from build123d import *

# Parameters (mm, degrees)
F1_DEPTH = 12.7
F3_DEPTH = 12.7
F5_D     = 16.002


with BuildPart() as f1:
    # F0 (on Front) → F1 (new body)
    with BuildSketch(Plane.XZ):
        with BuildLine():
            Line((0, 69.85), (0, 0))
            Line((0, 0), (15.67386, 0))
            Line((15.67386, 0), (16.004092, 12.86297))
            ThreePointArc((16.004092, 12.86297), (21.769188, 19.023198), (28.563172, 14.020547))
            ThreePointArc((28.563172, 14.020547), (28.702, 12.7), (28.563172, 11.379453))
            Line((28.563172, 11.379453), (28.563172, 0))
            Line((28.563172, 0), (44.704, 0))
            Line((44.704, 0), (44.704, 69.85))
            ThreePointArc((44.704, 69.85), (22.352, 92.202), (0, 69.85))
        make_face()
    extrude(amount=F1_DEPTH)

    # F2 (on face) → F3 (join)
    with BuildSketch(Plane.XZ.offset(12.7)):
        with BuildLine():
            Line((0, 69.85), (0, 44.45))
            Line((0, 44.45), (2.100821, 44.45))
            Line((2.100821, 44.45), (44.704, 44.45))
            Line((44.704, 44.45), (44.704, 69.85))
            ThreePointArc((44.704, 69.85), (22.352, 92.202), (0, 69.85))
        make_face()
    extrude(amount=F3_DEPTH)

    # F5 (through all)
    with Locations(Plane.XZ.offset(25.4)):
        with Locations((22.352, 69.85)):
            Hole(F5_D / 2)


solid = f1.part
Could you check a few things on this model? Use its own coordinates, in mm. A direction names the side the tool comes from. Round coordinates to 2 decimals unless told otherwise and drop trailing zeros. Order: outer loops, then holes, each group sorted by start corner. A loop starts at its lowest first (then second) coordinate and runs counter-clockwise, first axis right, second up.
(1) If we mould it in two halves opening along X, with no side actions, what happens to faces 1 (the flat face through (17, -25.4, 63)), 2 (the flat face through (0, -10, 43)), 3 (the flat face through (28.563, -6, 6))? For each: released by +X, released by -X, zero draft, split by the parting line, or undercut.
Response values:
face 1: zero draft
face 2: released by -X
face 3: undercut
(2) Imagine slicing it at A-A (z = 72). Write out the boundary of the cut face in (x, y), plus the area to 3 significant figures.
Response values:
outline: (0.1, -25.4) - (14.65, -25.4) - (14.65, 0) - (0.1, 0) - close; (30.06, -25.4) - (44.6, -25.4) - (44.6, 0) - (30.06, 0) - close
area: 739 mm2
(3) Imagine slicing it at D-D (y = -14.5). Write out the boundary of the cut face in (x, z).
Response values:
outline: (0, 44.45) - (44.7, 44.45) - (44.7, 69.85) arc R22.35 ccw to (0, 69.85) - close; hole circle Ø16 at (22.35, 69.85)
(4) Imagine slicing it at B-B (y = -6.5). Write out the boundary of the cut face in (x, z).
Response values:
outline: (0, 0) - (15.67, 0) - (16, 12.86) arc R6.35 cw to (28.56, 14.02) arc R6.35 cw to (28.56, 11.38) - (28.56, 0) - (44.7, 0) - (44.7, 69.85) arc R22.35 ccw to (0, 69.85) - close; hole circle Ø16 at (22.35, 69.85)
(5) I'm going to push flat-ended pins straight in: pin 1 (3 mm diameter, centred on x = 17, y = -14, fed in from +Z); pin 2 (6.5 mm diameter, centred on x = 27.5, y = -18, fed in from -Z); pin 3 (9.5 mm diameter, centred on x = 22.352, z = 69.85, fed in from +Y). Where does each tip first touch, or does it pass through?
Response values:
pin 1: stops at z = 91.87
pin 2: stops at z = 44.45
pin 3: passes through
(6) Imagine slicing it at C-C (x = 24.5). Write out the boundary of the cut face in (y, z), plus the area to 3 significant figures.
Response values:
outline: (-25.4, 44.45) - (-12.7, 44.45) - (-12.7, 18.68) - (0, 18.68) - (0, 62.14) - (-25.4, 62.14) - close; (-25.4, 77.56) - (0, 77.56) - (0, 92.1) - (-25.4, 92.1) - close
area: 1,150 mm2
(7) Please list where these lines run through material, in increasing order: line 1 along Y through (x, z) = (37, 38.5); line 2 along Z through (x, y) = (26.5, -16.25); line 3 along X through (y, z) = (-4, 18).
Response values:
line 1: y = -12.7 to 0
line 2: z = 44.45 to 63.01, 76.69 to 91.81
line 3: x = 0 to 18.85, 25.85 to 44.7
(8) Which directions (+Z, -Z, +X, -X, +Y, -Y) give clear straight access to the entire face, cutting with the end or side of a thin tool? Please do faces 4 (the flat face through (37, -6, 0)), 5 (the flat face through (22, -12.7, 23)).
Response values:
face 4: -Z, +X, -X, +Y, -Y
face 5: -Z, +X, -X, -Y
